Geometry: see drawing. Coordinates: mm, zero at the bounding-box minimum. A direction names the side the tool comes from. Round coordinates to 2 decimals unless told otherwise and drop trailing zeros. Loops run counter-clockwise (first coordinate to the right, second up) from the corner with the lowest first, then second, coordinate; pieces in that order, holes last. Notation, with made-up numbers: (-5.75, 70.5) -> (30.25, 70.5) arc R24 cw to (30.25, 88.5) -> close; hole circle Ø6 at (76, 60). An arc over 180 degrees is marked (long way). Answer in a Markdown table with one row per item.
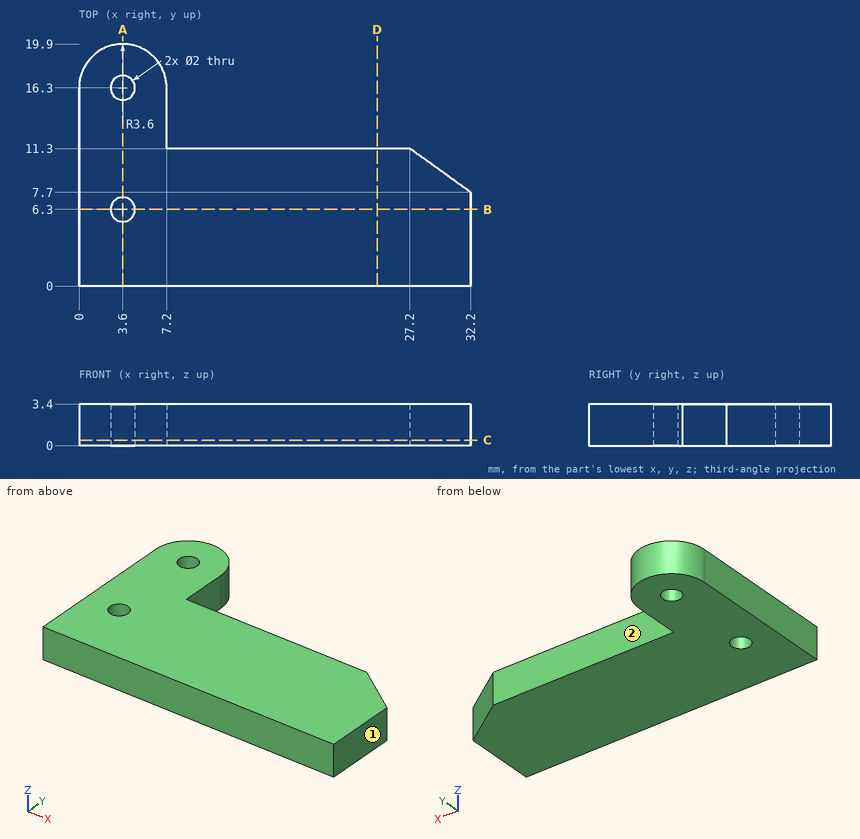
Item 1: Ray query, L1, parallel to Y at x = 3.6, z = 2.6; L2, parallel to Y at x = 4.5, z = 1.45; L3, parallel to X at y = 14, z = 3.1. Return the intervals inside material, ascending.
Ans:
| item | result |
|---|---|
| L1 | 0 to 5.3, 7.3 to 15.3, 17.3 to 19.9 |
| L2 | 0 to 5.86, 6.74 to 15.86, 16.74 to 19.79 |
| L3 | 0 to 7.2 |
Item 2: Section query C-C, the plane z = 0.45. Output: boundary loops of the cut face in (x, y).
Ans:
| item | result |
|---|---|
| outline | (0, 0) -> (32.2, 0) -> (32.2, 7.7) -> (27.2, 11.3) -> (7.2, 11.3) -> (7.2, 16.3) arc R3.6 ccw to (0, 16.3) -> close; hole circle Ø2 at (3.6, 6.3); hole circle Ø2 at (3.6, 16.3) |
Item 3: Section query A-A, the plane x = 3.6. Output: boundary loops of the cut face in (y, z).
Ans:
| item | result |
|---|---|
| outline | (0, 0) -> (5.3, 0) -> (5.3, 3.4) -> (0, 3.4) -> close; (7.3, 0) -> (15.3, 0) -> (15.3, 3.4) -> (7.3, 3.4) -> close; (17.3, 0) -> (19.9, 0) -> (19.9, 3.4) -> (17.3, 3.4) -> close |
Item 4: Section query B-B, the plane y = 6.3. Output: boundary loops of the cut face in (x, z).
Ans:
| item | result |
|---|---|
| outline | (0, 0) -> (2.6, 0) -> (2.6, 3.4) -> (0, 3.4) -> close; (4.6, 0) -> (32.2, 0) -> (32.2, 3.4) -> (4.6, 3.4) -> close |
Item 5: Set-up query: the marked faces 1 and 2. Return all of +Z, -Z, +X, -X, +Y, -Y with unobstructed straight access to the full face (end or side cutting, diameter ignored); none if empty.
Ans:
| item | result |
|---|---|
| face 1 | +Z, -Z, +X, +Y, -Y |
| face 2 | +Z, -Z, +X, +Y |
Item 6: Section query D-D, the plane x = 24.5. Output: boundary loops of the cut face in (y, z), and give its area (3 significant figures).
Ans:
| item | result |
|---|---|
| outline | (0, 0) -> (11.3, 0) -> (11.3, 3.4) -> (0, 3.4) -> close |
| area | 38.4 mm2 |
Item 7: First-contact query: P1, Ø1.8, axis at x = 3.6, y = 16.3, coming from the -Z side; P2, Ø1, axis at y = 13, z = 1, coming from the +X side. Flat tips, straight axial feed; report the tip coordinate or a pass-through.
Ans:
| item | result |
|---|---|
| P1 | through |
| P2 | x = 7.2 |
